For this review, take the finished solid that the model builds, in its own axes (mm). A direction names the side the tool comes from. Give positions to 0.01 mm unless a question says otherwise; leave off trailing zeros. Order: outer loops, then holes, each group sorted by start corner. A loop starts at its lowest first (then second) coordinate and runs counter-clockwise, first axis right, second up.
from build123d import *
from OCP.BRepFilletAPI import BRepFilletAPI_MakeChamfer

# Parameters (mm, degrees)
BOSS_EXTRUDE1_DEPTH     = 33
CUT_EXTRUDE2_DEPTH      = 70.814038703
CUT_EXTRUDE2_DEPTH_BACK = 70.814038703
SKETCH5_R               = 16.5
SKETCH5_R_2             = 4.25
BOSS_EXTRUDE2_DEPTH     = 15
CHAMFER1_SIZE           = 3
CHAMFER1_SIZE_2         = 3.575260778
CUT_EXTRUDE_THIN1_START = -15
SKETCH6_W               = 1
SKETCH6_H               = 51.277142369
CUT_EXTRUDE_THIN1_DEPTH = 15
CHAMFER2_SIZE           = 5
CHAMFER2_SIZE2          = 5.958767963


with BuildPart() as part:
    # Sketch1 → Boss-Extrude1 (new body)
    with BuildSketch(Plane.XY):
        Polygon((0, 0), (0, 40), (41, 40), (41, 0), (44, 0), (44, 43), (-3, 43), (-3, 0), align=None)
    extrude(amount=BOSS_EXTRUDE1_DEPTH)

    # Sketch4 → Cut-Extrude2 (cut, two sides: drawn at the far end of the back side and taken through both)
    with BuildSketch(Plane(origin=(0, 0, 0), x_dir=(0, 0, -1), z_dir=(1, 0, 0)).offset(-CUT_EXTRUDE2_DEPTH_BACK)):
        with BuildLine():
            Line((-21.5, 22.5), (-11.5, 22.5))
            ThreePointArc((-11.5, 22.5), (-9, 20), (-11.5, 17.5))
            Line((-11.5, 17.5), (-21.5, 17.5))
            ThreePointArc((-21.5, 17.5), (-24, 20), (-21.5, 22.5))
        make_face()
    extrude(amount=CUT_EXTRUDE2_DEPTH + CUT_EXTRUDE2_DEPTH_BACK, mode=Mode.SUBTRACT)

    # Sketch5 → Boss-Extrude2 (add)
    with BuildSketch(Plane(origin=(0, 43, 0), x_dir=(1, 0, 0), z_dir=(0, 1, 0))):
        with Locations(Location((20.5, -16.5, 0), (0, 0, 270))):
            Circle(SKETCH5_R)
        with Locations(Location((20.5, -16.5, 0), (0, 0, 270))):
            Circle(SKETCH5_R_2, mode=Mode.SUBTRACT)
    extrude(amount=BOSS_EXTRUDE2_DEPTH)

    # Chamfer1
    # the kernel refuses this chamfer: 3.575260778, 3 mm, written as the material it adds along each edge
    with BuildSketch(Plane(origin=(20.5, 43, 16.5), x_dir=(0, 0, -1), z_dir=(1, 0, 0))) as chamfer1_piece_1_section:
        Polygon((16.5 + CHAMFER1_SIZE, 0), (16.5, CHAMFER1_SIZE_2), (16.5, 0), align=None)
    chamfer1_piece_1 = revolve(axis=Axis((20.5, 43, 16.5), (0, 1, 0)), revolution_arc=180, mode=Mode.PRIVATE)
    chamfer1_piece_1 = split(chamfer1_piece_1, bisect_by=Plane(origin=(2.547299358, 44.747941515, 0), z_dir=(0, 0, 1)), keep=Keep.TOP, mode=Mode.PRIVATE)
    chamfer1_piece_1 = split(chamfer1_piece_1, bisect_by=Plane(origin=(2.547299358, 44.747941515, 33), z_dir=(0, 0, -1)), keep=Keep.TOP, mode=Mode.PRIVATE)
    add(chamfer1_piece_1)
    with BuildSketch(Plane(origin=(20.5, 43, 16.5), x_dir=(0, 0, 1), z_dir=(-1, 0, 0))) as chamfer1_piece_2_section:
        Polygon((16.5 + CHAMFER1_SIZE, 0), (16.5, CHAMFER1_SIZE_2), (16.5, 0), align=None)
    chamfer1_piece_2 = revolve(axis=Axis((20.5, 43, 16.5), (0, 1, 0)), revolution_arc=180, mode=Mode.PRIVATE)
    chamfer1_piece_2 = split(chamfer1_piece_2, bisect_by=Plane(origin=(38.452700642, 44.747941515, 0), z_dir=(0, 0, 1)), keep=Keep.TOP, mode=Mode.PRIVATE)
    chamfer1_piece_2 = split(chamfer1_piece_2, bisect_by=Plane(origin=(38.452700642, 44.747941515, 33), z_dir=(0, 0, -1)), keep=Keep.TOP, mode=Mode.PRIVATE)
    add(chamfer1_piece_2)

    # Sketch6 → Cut-Extrude-Thin1 (cut)
    with BuildSketch(Plane(origin=(0, 58, 0), x_dir=(1, 0, 0), z_dir=(0, 1, 0)).offset(CUT_EXTRUDE_THIN1_START)):
        with Locations((20.5, 9.138571185)):
            Rectangle(SKETCH6_W, SKETCH6_H)
    extrude(amount=CUT_EXTRUDE_THIN1_DEPTH, mode=Mode.SUBTRACT)

    # Chamfer2: one chamfer whose edges measure the first distance from different faces: ONE call of the kernel's chamfer builder (chamfer() names one face for all edges)
    chamfer2_edges_1 = [part.edges().sort_by_distance(p)[0] for p in [
        (-1.5, 0, 0),
        (42.5, 0, 0),
    ]]
    chamfer2_side_1 = [part.faces().sort_by_distance(p)[0] for p in [
        (25.936545793, 44.827539599, 0),
    ]]
    chamfer2_edges_2 = [part.edges().sort_by_distance(p)[0] for p in [
        (42.5, 0, 33),
    ]]
    chamfer2_side_2 = [part.faces().sort_by_distance(p)[0] for p in [
        (42.5, 0, 16.5),
    ]]
    chamfer2_edges_3 = [part.edges().sort_by_distance(p)[0] for p in [
        (-1.5, 0, 33),
    ]]
    chamfer2_side_3 = [part.faces().sort_by_distance(p)[0] for p in [
        (-1.5, 0, 16.5),
    ]]
    chamfer2 = BRepFilletAPI_MakeChamfer(part.part.solid().wrapped)
    for e in chamfer2_edges_1:
        chamfer2.Add(CHAMFER2_SIZE, CHAMFER2_SIZE2, e.wrapped, chamfer2_side_1[0].wrapped)  # the first distance lies on this face
    for e in chamfer2_edges_2:
        chamfer2.Add(CHAMFER2_SIZE, CHAMFER2_SIZE2, e.wrapped, chamfer2_side_2[0].wrapped)  # the first distance lies on this face
    for e in chamfer2_edges_3:
        chamfer2.Add(CHAMFER2_SIZE, CHAMFER2_SIZE2, e.wrapped, chamfer2_side_3[0].wrapped)  # the first distance lies on this face
    add(Compound.cast(chamfer2.Shape()), mode=Mode.REPLACE)


solid = part.part
1) Tool access review of faces 1 (the face through (42.479, 3.021, 30.535)), 2 (the face through (42, 20, 24)), 3 (the face through (20, 40, 16)), 4 (the face through (19, 41, 0)), 5 (the face through (20, 43, 15)): name each direction out of +Z, -Z, +X, -X, +Y, -Y from which nothing blocks a thin tool from reaching the whole face with its end or side.
Answer sheet:
face 1: +Z, +X, -X, -Y
face 2: +X, -X
face 3: +Z, -Z, -Y
face 4: -Z, +X, -X, +Y, -Y
face 5: +Y
2) We need section B-B on y = 20. Give the boundary of the cut face in (x, z).
Answer sheet:
outline: (-3, 0) - (0, 0) - (0, 9) - (-3, 9) - close; (-3, 24) - (0, 24) - (0, 33) - (-3, 33) - close; (41, 0) - (44, 0) - (44, 9) - (41, 9) - close; (41, 24) - (44, 24) - (44, 33) - (41, 33) - close
3) To check wall thickness, follow line 1 (X direction, y = 29.5, z = 25.5); line 2 (Y direction, x = 40, z = 29.5); line 3 (Y direction, x = 6.5, z = 22). State the ranges of each line that lie inside material, in increasing order.
Answer sheet:
line 1: x = -3 to 0, 41 to 44
line 2: y = 40 to 43
line 3: y = 40 to 58
4) We need section C-C on y = 38. Give the boundary of the cut face in (x, z).
Answer sheet:
outline: (-3, 0) - (0, 0) - (0, 33) - (-3, 33) - close; (41, 0) - (44, 0) - (44, 33) - (41, 33) - close
5) Draft analysis for pull direction Z (two halves, no side actions). For faces 6 (the face through (-1.521, 2.465, 3.021)), 7 (the face through (-2, 20, 24)), 8 (the face through (0.7, 43, 16.3)), 9 (the face through (42, 22.5, 17)), state which applies: +Z half, -Z half, draft (parallel to the pull), parting line (faces both ways), or undercut.
Answer sheet:
face 6: -Z half
face 7: undercut
face 8: draft
face 9: undercut
6) We need section D-D on y = 53. Give the boundary of the cut face in (x, z), then the cut area to 3 significant figures.
Answer sheet:
outline: (20, 0.01) - (20, 12.28) arc R4.25 cw (long way) to (21, 12.28) - (21, 0.01) arc R16.5 ccw (long way) to start
area: 786 mm2
7) Clearance check with flat-ended pins moving along their axes: pin 1 (0.9 mm diameter, centred on x = -1.5, z = 19, fed in from +Y); pin 2 (10 mm diameter, centred on x = 11.5, z = 14, fed in from -Y); pin 3 (6 mm diameter, centred on x = 2, z = 13, fed in from +Y); pin 4 (3 mm diameter, centred on y = 45, z = 17.5, fed in from -X). State where each tip first meets the part, or that it passes through.
Answer sheet:
pin 1: stops at y = 43
pin 2: stops at y = 40
pin 3: stops at y = 58
pin 4: stops at x = 1.44
8) We need section A-A on z = 16.5. Give the boundary of the cut face in (x, y).
Answer sheet:
outline: (-3, 0) - (0, 0) - (0, 17.5) - (-3, 17.5) - close; (-3, 22.5) - (0, 22.5) - (0, 40) - (41, 40) - (41, 22.5) - (44, 22.5) - (44, 43) - (40, 43) - (37, 46.58) - (37, 58) - (24.75, 58) - (24.75, 43) - (16.25, 43) - (16.25, 58) - (4, 58) - (4, 46.58) - (1, 43) - (-3, 43) - close; (41, 0) - (44, 0) - (44, 17.5) - (41, 17.5) - close
